For this review, take the finished solid that the model builds, in its own axes (mm). A direction names the side the tool comes from. Round coordinates to 2 decimals unless told otherwise and drop trailing zeros. Order: outer loops, then holes, each group sorted by start corner. A loop starts at its lowest first (then second) coordinate and runs counter-clockwise, first axis right, second up. Notation, with made-up numbers: M 33,22 L 76,22 A12 cw 76,26 Z; hole C 35,73 d3. An arc over 180 degrees is marked long. Answer as a JSON object with one key per item and string values.
from build123d import *

# Parameters (mm, degrees)
F0_W     = 40
F0_H     = 40
F1_DEPTH = 40
F4_DEPTH = 7
F6_REACH = 50.3537618041
F8_REACH = 50.3537618041


with BuildPart() as f1:
    # F0 (on Front) → F1 (new body)
    with BuildSketch(Plane.XZ):
        with Locations((20, 20)):
            Rectangle(F0_W, F0_H)
    extrude(amount=F1_DEPTH)

    # F3 (on offset) → F4 (cut, symmetric)
    with BuildSketch(Plane.XZ.offset(20)):
        Polygon((0, 40), (0, 17.3205080757), (10, 20), (30, 20), (40, 17.3205080757), (40, 40), align=None)
    extrude(amount=F4_DEPTH, both=True, mode=Mode.SUBTRACT)

    f6_end = Plane(origin=(5, -20, 18.6602540378), x_dir=(0.9659258263, 0, 0.2588190451), z_dir=(-0.2588190451, 0, 0.9659258263))
    # F5 (on face) → F6 (cut, up to a plane its end follows)
    with BuildSketch(Plane.XY.offset(40)):
        Polygon((10, -13), (0, -10.3205080757), (0, -13), align=None)
        Polygon((0, -27), (0, -29.6794919243), (10, -27), align=None)
    f6_long = extrude(amount=-F6_REACH, mode=Mode.PRIVATE)
    add(split(f6_long, bisect_by=f6_end, keep=Keep.TOP, mode=Mode.PRIVATE), mode=Mode.SUBTRACT)

    f8_end = Plane(origin=(35, -20, 18.6602540378), x_dir=(0.9659258263, 0, -0.2588190451), z_dir=(0.2588190451, 0, 0.9659258263))
    # F7 (on face) → F8 (cut, up to a plane its end follows)
    with BuildSketch(Plane.XY.offset(40)):
        Polygon((40, -10.3205080757), (30, -13), (40, -13), align=None)
        Polygon((40, -27), (30, -27), (40, -29.6794919243), align=None)
    f8_long = extrude(amount=-F8_REACH, mode=Mode.PRIVATE)
    add(split(f8_long, bisect_by=f8_end, keep=Keep.TOP, mode=Mode.PRIVATE), mode=Mode.SUBTRACT)


solid = f1.part
1) Add section B-B on y = -22. State the section outline as (x, z) points, and give its area (3 significant figures).
Geometry check:
{"outline": "M 0,0 L 40,0 L 40,17.32 L 30,20 L 10,20 L 0,17.32 Z", "area": "773 mm²"}
2) Add section D-D on x = 17. State the section outline as (y, z) points, and give its area (3 significant figures).
Geometry check:
{"outline": "M -40,0 L 0,0 L 0,40 L -13,40 L -13,20 L -27,20 L -27,40 L -40,40 Z", "area": "1,320 mm²"}
3) Add section A-A on z = 34.5. State the section outline as (x, y) points, and give its area (3 significant figures).
Geometry check:
{"outline": "M 0,-40 L 40,-40 L 40,-29.68 L 30,-27 L 10,-27 L 0,-29.68 Z; M 0,-10.32 L 10,-13 L 30,-13 L 40,-10.32 L 40,0 L 0,0 Z", "area": "986 mm²"}
4) For L1, parallel to Y at x = 14.5, z = 22; L2, parallel to Z at x = 19.5, y = -26; L3, parallel to Y at x = 2.5, z = 27, list the stretches that pass through material, from the lowest coordinate up.
Geometry check:
{"L1": "y = -40 to -27, -13 to 0", "L2": "z = 0 to 20", "L3": "y = -40 to -29.01, -10.99 to 0"}
5) Insertion check: P1, Ø1, axis at x = 5.5, y = -22, coming from the +Z side. The pin has a flat end and moves straight along its axis. Give the tip position at first contact, or say it passes through.
Geometry check:
{"P1": "stops at z = 18.93"}
6) Machinability: for faces 1 (the flat face through (4.93, -28.36, 28.82)), 2 (the flat face through (20, -13, 30)), 3 (the flat face through (35.07, -11.64, 28.82)), which of the approach directions +Z, -Z, +X, -X, +Y, -Y give a long, thin tool a straight path to every point of the face, cutting with its end or side? Answer none if there is none.
Geometry check:
{"face 1": "+Z, -X", "face 2": "+Z, +X, -X", "face 3": "+Z, +X"}
7) Mouldability with a two-part tool opening along Y and no side actions: class faces 4 (the flat face through (20, -40, 20)), 5 (the flat face through (20, -20, 0)), 6 (the flat face through (5.07, -11.68, 28.82)), 7 (the flat face through (20, 0, 20)) as +Y half, -Y half, draft (parallel to the pull), parting line (faces both ways), or undercut.
Geometry check:
{"face 4": "-Y half", "face 5": "draft", "face 6": "undercut", "face 7": "+Y half"}
8) Add section C-C on x = 35. State the section outline as (y, z) points, and give its area (3 significant figures).
Geometry check:
{"outline": "M -40,0 L 0,0 L 0,40 L -11.66,40 L -11.66,18.66 L -28.34,18.66 L -28.34,40 L -40,40 Z", "area": "1,240 mm²"}
